Input: part model. Units: mm. Frame: model coordinates. A direction names the side the tool comes from. Round coordinates to 2 decimals unless told otherwise and drop trailing zeros. Write each loop counter-clockwise with the first axis right and the second up, starting at its lowest first coordinate (ties: lowest second). Pieces come first, ordered by that corner, then holes. Notation, with made-up numbers: (50, 81) -> (76, 81) arc R27 ccw to (76, 112) -> close; hole circle Ø11 at (89.25, 46.5). An arc over 180 degrees is marked (long way). Write item = value, one per line.
Autodesk Inventor part; units mm, degrees
ref_plane "YZ Plane" through (0, 0, 0) normal (1, 0, 0) x (0, 1, 0)
ref_plane "XZ Plane" through (0, 0, 0) normal (0, 1, 0) x (-1, 0, 0)
ref_plane "XY Plane" through (0, 0, 0) normal (0, 0, 1) x (1, 0, 0)
sketch "草圖1" plane through (0, 0, 0) normal (0, 1, 0) x (-1, 0, 0)
  line L0 (2.5, 15) -> (-2.5, 15)
  line L1 (-2.5, 15) -> (-2.5, -15)
  line L2 (-2.5, -15) -> (2.5, -15)
  line L3 (2.5, -15) -> (2.5, 15)
  circle A0 centre (0, 12.5) radius 1.7
  circle A1 centre (0, 7.5) radius 1.7
  circle A2 centre (0, 2.5) radius 1.7
  circle A3 centre (0, -2.5) radius 1.7
  circle A4 centre (0, -7.5) radius 1.7
  circle A5 centre (0, -12.5) radius 1.7
  point P0 (0, 0)
  point P1 (2.5, 0)
  point P2 (0, 15)
  dimension "d0" = 5
  dimension "d1" = 30
  dimension "d2" = 3.4
  dimension "d3" = 2.5
  dimension "d4" = 2.5
  dimension "d7" = 5
extrude "擠出1" add sketch "草圖1" along normal blind 2 contours L3 L2 L1 L0 | A0 | A1 | A2 | A3 | A4 | A5
extrude "擠出2" cut sketch "草圖1" along normal blind 1.5 contours A0 | A1 | A2 | A3 | A4 | A5
sketch "草圖2" plane through (2.5, 0, 15) normal (1, 0, 0) x (0, 0, -1)
  line L0 (-1, 10) -> (31, 10)
  line L1 (31, 10) -> (31, 0)
  line L2 (31, 0) -> (-1, 0)
  line L3 (-1, 0) -> (-1, 10)
  line L4 (0, 0) -> (30, 0)
  line L5 (30, 9) -> (0, 9)
  line L6 (0, 9) -> (0, 1)
  line L7 (0, 1) -> (30, 1)
  line L8 (30, 1) -> (30, 9)
  point P0 (15, 0)
  point P1 (15, 10)
  point P2 (15, 0)
  point P3 (15, 0)
  dimension "d16" = 32
  dimension "d17" = 10
  dimension "d18" = 1
extrude "擠出3" add sketch "草圖2" along normal blind 1.5
properties part number "110033226_ipt_20_塔樓窗戶"
1) Cut plane C-C (z = 12). Return the cut outline in (x, y), and give its area (3 significant figures).
Solutions:
outline = (-2.5, 0) -> (-1.62, 0) -> (-1.62, 1.5) -> (1.62, 1.5) -> (1.62, 0) -> (4, 0) -> (4, 1) -> (2.5, 1) -> (2.5, 2) -> (-2.5, 2) -> close; (2.5, 9) -> (4, 9) -> (4, 10) -> (2.5, 10) -> close
area = 8.13 mm^2
2) First-contact query: P1, Ø0.8, axis at y = 1.5, z = 7.5, coming from the +X side; P2, Ø1, axis at x = 0, z = -13, coming from the -Y side; P3, Ø1, axis at x = 0, z = -8, coming from the +Y side. Flat tips, straight axial feed; report the tip coordinate or a pass-through.
Solutions:
P1 = 2.5
P2 = 1.5
P3 = 2
3) Cut plane B-B (x = 3). Return the cut outline in (y, z).
Solutions:
outline = (0, -16) -> (10, -16) -> (10, 16) -> (0, 16) -> close; hole (1, -15) -> (9, -15) -> (9, 15) -> (1, 15) -> close
4) Draft query along Y for faces 4 (the face through (2.5, 9.5, 0.1)), 5 (the face through (3, 5, -15)), 6 (the face through (0, 1.5, 13)). Return one class per face: +Y half, -Y half, draft (parallel to the pull), parting line (faces both ways), or undercut.
Solutions:
face_4 = draft
face_5 = undercut
face_6 = -Y half
5) Access query for faces 1 (the face through (0, 1.5, -2)), 2 (the face through (2.5, 1.5, 0.2)), 3 (the face through (0, 1, 15)). Directions: +Z, -Z, +X, -X, +Y, -Y. A direction counts if a zero-diameter tool reaches every point of the face in a straight line with its end or side. Return the directions, or none.
Solutions:
face_1 = -Y
face_2 = +X
face_3 = +Z, -X, +Y, -Y
6) Line query: L1, parallel to Y at x = 1.25, z = -10; L2, parallel to X at y = 1.5, z = -10.5; L3, parallel to Y at x = -0.25, z = 14. Output: solid intervals per line, ascending. Write a range as from..to.
Solutions:
L1 = 0..2
L2 = -2.5..2.5
L3 = 1.5..2
7) Cut plane D-D (x = 1). Return the cut outline in (y, z), and give its area (3 significant figures).
Solutions:
outline = (0, -15) -> (2, -15) -> (2, 15) -> (0, 15) -> (0, 13.87) -> (1.5, 13.87) -> (1.5, 11.13) -> (0, 11.13) -> (0, 8.87) -> (1.5, 8.87) -> (1.5, 6.13) -> (0, 6.13) -> (0, 3.87) -> (1.5, 3.87) -> (1.5, 1.13) -> (0, 1.13) -> (0, -1.13) -> (1.5, -1.13) -> (1.5, -3.87) -> (0, -3.87) -> (0, -6.13) -> (1.5, -6.13) -> (1.5, -8.87) -> (0, -8.87) -> (0, -11.13) -> (1.5, -11.13) -> (1.5, -13.87) -> (0, -13.87) -> close
area = 35.3 mm^2
8) Cut plane A-A (y = 5.5). Return the cut outline in (x, z).
Solutions:
outline = (2.5, -16) -> (4, -16) -> (4, -15) -> (2.5, -15) -> close; (2.5, 15) -> (4, 15) -> (4, 16) -> (2.5, 16) -> close
